Check sheet for the modelled part. Datum: model origin and axes. Units: mm. A direction names the side the tool comes from. Round coordinates to 2 decimals unless told otherwise and drop trailing zeros. Order: outer loops, then holes, each group sorted by start corner. A loop starts at its lowest first (then second) coordinate and runs counter-clockwise, first axis right, second up.
Q1. Cross-section at B-B on z = 15.24. Record the cut outline in (x, y).
Q2. Scan lines: probe 1 along X at (y, z) = (65.6, 21.59); probe 2 along X at (y, z) = (66.05, 15.24); probe 3 along Z at (x, y) = (38.1, 65.9). Record each from-to range of solid material in increasing order.
Q3. Cross-section at A-A on x = 38.1. Record the cut outline in (y, z).
Q4. Set-up check for faces 1 (the flat face through (47, 85, 14)), 2 (the flat face through (34.32, 66.05, 22.7)), 3 (the cylindrical face through (52.345, 66.004, 23.275)): record each of +Z, -Z, +X, -X, +Y, -Y from which the full face is reachable in a straight line by a thin tool's end or side.
Q5. Mould release check, pull along X, two halves, no side actions. Record for faces 4 (the cylindrical face through (37.22, 66, 13.13)), 5 (the flat face through (47, 86, -3.048)), 6 (the flat face through (68.58, 76, 6)): +X half, -X half, draft (parallel to the pull), parting line (faces both ways), or undercut.
Q6. Cross-section at D-D on x = 56.5. Record the cut outline in (y, z), then the cut area to 3 significant figures.
Q7. Cross-section at C-C on y = 78.5. Record the cut outline in (x, z), then the cut area to 3 significant figures.
Q8. Depth check by flat-ended pin: P1, Ø1.5, axis at x = 39.5, z = 5.5, coming from the +Y side; P2, Ø8, axis at x = 44.5, y = 94.5, coming from the +Z side; P3, Ø5.5, axis at x = 38.1, z = 15.24, coming from the +Y side. Enter the tip coordinate at first touch or a pass-through.
from build123d import *

# Parameters (mm, degrees)
PAD032_DEPTH    = 43.18
SKETCH068_R     = 2.286
POCKET031_DEPTH = 5.08
SKETCH069_R     = 2.286
POCKET032_DEPTH = 4.318


with BuildPart() as part:
    # Sketch067 → Pad032 (new body)
    with BuildSketch(Plane.YZ):
        Polygon((0, 0), (0, 33.02), (44.45, 0), align=None)
    extrude(amount=PAD032_DEPTH)

    # Sketch068 (on Face1 of Pad032) → Pocket031 (cut)
    with BuildSketch(Plane(origin=(0, 0, 0), x_dir=(0, 0, -1), z_dir=(0, -1, 0))):
        with Locations((-18.288, 12.7)):
            Circle(SKETCH068_R)
        with Locations((-24.638, 25.4)):
            Circle(SKETCH068_R)
    extrude(amount=-POCKET031_DEPTH, mode=Mode.SUBTRACT)

    # Sketch069 (on Face5 of Pocket031) → Pocket032 (cut)
    with BuildSketch(Plane(origin=(0, 15.8065228827, 21.2780115729), x_dir=(0, -0.802743848, 0.5963240013), z_dir=(0, 0.5963240013, 0.802743848))):
        with Locations((13.3406185242, 34.29)):
            Circle(SKETCH069_R)
        with Locations((13.3406185242, 8.89)):
            Circle(SKETCH069_R)
        with Locations((-24.7593814758, 34.29)):
            Circle(SKETCH069_R)
        with Locations((-24.7593814758, 8.89)):
            Circle(SKETCH069_R)
    extrude(amount=-POCKET032_DEPTH, mode=Mode.SUBTRACT)


with BuildPart() as part_1:
    # Body024 placement: moved
    add(part.part.moved(Location((25.4, 63.5, -3.048))))


solid = part_1.part
Results found:
1. outline: (25.4, 63.5) - (35.81, 63.5) - (35.81, 68.58) - (40.39, 68.58) - (40.39, 63.5) - (68.58, 63.5) - (68.58, 83.33) - (25.4, 83.33) - close
2. probe 1: x = 25.4 to 48.51, 53.09 to 68.58
2. probe 2: x = 25.4 to 35.81, 40.39 to 68.58
2. probe 3: z = -3.05 to 12.95, 17.53 to 28.19
3. outline: (63.5, -3.05) - (107.95, -3.05) - (63.5, 29.97) - (63.5, 17.53) - (68.58, 17.53) - (68.58, 12.95) - (63.5, 12.95) - close
4. face 1: +Z, +X, -X, +Y
4. face 2: none
4. face 3: -Y
5. face 4: undercut
5. face 5: draft
5. face 6: +X half
6. outline: (63.5, -3.05) - (107.95, -3.05) - (63.5, 29.97) - close
6. area: 734 mm2
7. outline: (25.4, -3.05) - (68.58, -3.05) - (68.58, 18.83) - (25.4, 18.83) - close
7. area: 945 mm2
8. P1: stops at y = 97.45
8. P2: stops at z = 9.91
8. P3: stops at y = 87.03
